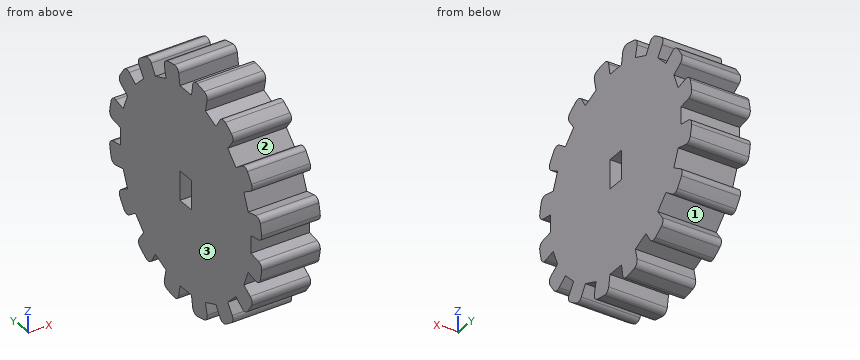
```python
from build123d import *

# Parameters (mm, degrees)
SKETCH4_W                = 5
SKETCH4_H                = 3
CUT_EXTRUDE2_DEPTH       = 10
CUT_EXTRUDE3_DEPTH       = 10
FILLET1_R                = 1
CIRPATTERN1_COUNT        = 16
FILLET1_OF_CIRPATTERN1_R = 1


with BuildPart() as part:
    # Sketch1 → Revolve1 (revolve)
    with BuildSketch(Plane.XY):
        Polygon((0, 0), (-10, 0), (-10, 5), (-10, 10), (-10, 20), (0, 20), (0, 5), align=None)
    revolve(axis=Axis((0, 0, 0), (-1, 0, 0)))

    # Sketch4 → Cut-Extrude2 (cut)
    with BuildSketch(Plane.ZY.offset(10)):
        Rectangle(SKETCH4_W, SKETCH4_H)
    extrude(amount=-CUT_EXTRUDE2_DEPTH, mode=Mode.SUBTRACT)

    # Sketch5 → Cut-Extrude3 (cut)
    with BuildSketch(Plane(origin=(0, 0, 0), x_dir=(0, 0, -1), z_dir=(1, 0, 0))):
        Polygon((-2.502016427, 23), (2.502016427, 23), (1.501758676, 17), (-1.501758676, 17), align=None)
    cut_extrude3 = extrude(amount=-CUT_EXTRUDE3_DEPTH, mode=Mode.SUBTRACT)

    # Fillet1
    fillet1_edges = [part.edges().sort_by_distance(p)[0] for p in [
        (-5, 19.90120888, -1.985418121),
        (-5, 19.90120888, 1.985418121),
    ]]
    fillet(fillet1_edges, radius=FILLET1_R)

    # CirPattern1: Cut-Extrude3 ×16 about axis
    cirpattern1_axis = Axis((0, 0, 0), (1, 0, 0))
    for i in range(1, CIRPATTERN1_COUNT):
        add(cut_extrude3.rotate(cirpattern1_axis, i * 360 / CIRPATTERN1_COUNT), mode=Mode.SUBTRACT)

    # Fillet1 of CirPattern1
    fillet1_of_cirpattern1_edges = [part.edges().sort_by_distance(p)[0] for p in [
        (-5, 19.146106178, 5.781575757),
        (-5, 17.626532935, 9.450150088),
        (-5, 15.47618237, 12.668377136),
        (-5, 12.668377136, 15.47618237),
        (-5, 9.450150088, 17.626532935),
        (-5, 5.781575757, 19.146106178),
        (-5, 1.985418121, 19.90120888),
        (-5, -1.985418121, 19.90120888),
        (-5, -5.781575757, 19.146106178),
        (-5, -9.450150088, 17.626532935),
        (-5, -12.668377136, 15.47618237),
        (-5, -15.47618237, 12.668377136),
        (-5, -17.626532935, 9.450150088),
        (-5, -19.146106178, 5.781575757),
        (-5, -19.90120888, 1.985418121),
        (-5, -19.90120888, -1.985418121),
        (-5, -19.146106178, -5.781575757),
        (-5, -17.626532935, -9.450150088),
        (-5, -15.47618237, -12.668377136),
        (-5, -12.668377136, -15.47618237),
        (-5, -9.450150088, -17.626532935),
        (-5, -5.781575757, -19.146106178),
        (-5, -1.985418121, -19.90120888),
        (-5, 1.985418121, -19.90120888),
        (-5, 5.781575757, -19.146106178),
        (-5, 9.450150088, -17.626532935),
        (-5, 12.668377136, -15.47618237),
        (-5, 15.47618237, -12.668377136),
        (-5, 17.626532935, -9.450150088),
        (-5, 19.146106178, -5.781575757),
    ]]
    fillet(fillet1_of_cirpattern1_edges, radius=FILLET1_OF_CIRPATTERN1_R)


solid = part.part
```
Geometry check sheet. Reference: the model listing, model coordinates, mm. Face numbers are marked on the shaded views. Coordinates: 2 decimals unless noted, no trailing zeros. Answer in a Markdown table with one row per item. Add a question column.
1. Gauge pin test, flat ends, axial feed: pin 1 Ø3.5 at (x, z) = (-7.5, -0.5) entering from +Y; pin 2 Ø3.5 at (x, y) = (-6, -0.5) entering from -Z; pin 3 Ø1.5 at (x, z) = (-3, -12.5) entering from +Y; pin 4 Ø12 at (y, z) = (-13, -13.5) entering from +X. Record the tip position at first contact, or that the pin passes through.
2. Draft check along Y on the marked faces 1, 2 and 3. Enter one of: +Y half, -Y half, draft (parallel to the pull), parting line (faces both ways), or undercut.
3. Material ranges on L1, parallel to Z at x = -7, y = 1; L2, parallel to Z at x = -2, y = 12; L3, parallel to Y at x = -1.75, z = 2, recorded low to high. Write a range as [from, to].
Data:
| question | item | result |
|---|---|---|
| 1 | pin 1 | stops at y = 19.62 |
| 1 | pin 2 | stops at z = -19.62 |
| 1 | pin 3 | stops at y = 16.18 |
| 1 | pin 4 | stops at x = 0 |
| 2 | face 1 | undercut |
| 2 | face 2 | undercut |
| 2 | face 3 | draft |
| 3 | L1 | z = [-17, -2.5], [2.5, 17] |
| 3 | L2 | z = [-15.99, -14.54], [-12.04, 12.04], [14.54, 15.99] |
| 3 | L3 | y = [-19.37, -1.5], [1.5, 19.37] |
